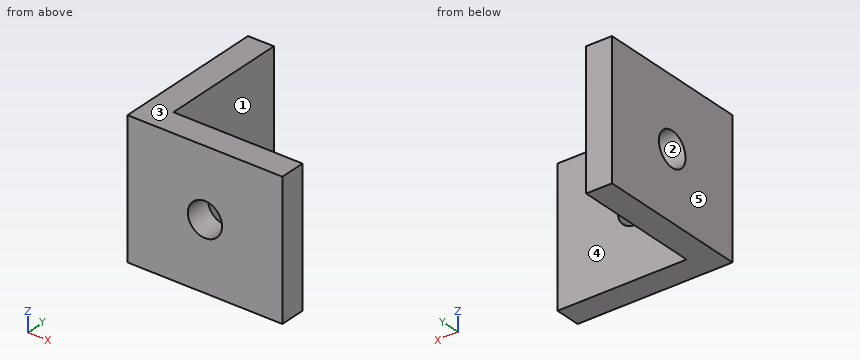
from build123d import *

# Parameters (mm, degrees)
BODY_DEPTH   = 33.27
SKETCH2_R    = 4.2
HOLESX_DEPTH = 6.35
SKETCH3_R    = 4.2
HOLESY_DEPTH = 6.35


with BuildPart() as part:
    # Sketch1 → Body (new body)
    with BuildSketch(Plane.XY.offset(-16.635)):
        Polygon((0, 0), (38.1, 0), (38.1, 6.35), (6.35, 6.35), (6.35, 38.1), (0, 38.1), align=None)
    extrude(amount=BODY_DEPTH)

    # Sketch2 → HolesX (cut)
    with BuildSketch(Plane(origin=(0, 6.35, 0), x_dir=(1, 0, 0), z_dir=(0, 1, 0))):
        with Locations(Location((19.05, 0, 0), (0, 0, 270))):
            Circle(SKETCH2_R)
    extrude(amount=-HOLESX_DEPTH, mode=Mode.SUBTRACT)

    # Sketch3 → HolesY (cut)
    with BuildSketch(Plane(origin=(6.35, 0, 0), x_dir=(0, 0, -1), z_dir=(1, 0, 0))):
        with Locations((0, 19.05)):
            Circle(SKETCH3_R)
    extrude(amount=-HOLESY_DEPTH, mode=Mode.SUBTRACT)


solid = part.part
Geometry check sheet. Reference: the model listing, model coordinates, mm. Face numbers are marked on the shaded views. A direction names the side the tool comes from. Coordinates: 2 decimals unless noted, no trailing zeros. Order: outer loops, then holes, each group sorted by start corner. A loop starts at its lowest first (then second) coordinate and runs counter-clockwise, first axis right, second up. Notation, with made-up numbers: (82.25, 74.25) - (94.25, 74.25) arc R17 ccw to (94.25, 89.25) - close; hole circle Ø3 at (33, 65.5). An arc over 180 degrees is marked (long way). One line per item, written item: value.
(1) Sectioned sample at C-C (z = 0). Enter the section's corners in (x, y), and give its area (3 significant figures).
Data:
outline: (0, 0) - (14.85, 0) - (14.85, 6.35) - (6.35, 6.35) - (6.35, 14.85) - (0, 14.85) - close; (0, 23.25) - (6.35, 23.25) - (6.35, 38.1) - (0, 38.1) - close; (23.25, 0) - (38.1, 0) - (38.1, 6.35) - (23.25, 6.35) - close
area: 337 mm^2
(2) Release check for a two-part mould opening along Z. For the marked faces 1, 2 and 3 record: +Z half, -Z half, draft (parallel to the pull), parting line (faces both ways), or undercut.
Data:
face 1: draft
face 2: undercut
face 3: +Z half
(3) Sectioned sample at A-A (y = 19.05). Enter the section's corners in (x, z) (3 decimals).
Data:
outline: (0, -16.635) - (6.35, -16.635) - (6.35, -4.2) - (0, -4.2) - close; (0, 4.2) - (6.35, 4.2) - (6.35, 16.635) - (0, 16.635) - close
(4) Thickness scan on probe 1 along X at (y, z) = (2.5, 0); probe 2 along Z at (x, y) = (1, 19) (3 decimals). Record the ranges inside material, lowest first. Write a range as from..to.
Data:
probe 1: x = 0..14.85, 23.25..38.1
probe 2: z = -16.635..-4.2, 4.2..16.635
(5) Sectioned sample at D-D (y = 7). Enter the section's corners in (x, z) (3 decimals).
Data:
outline: (0, -16.635) - (6.35, -16.635) - (6.35, 16.635) - (0, 16.635) - close
(6) Access from +Z, -Z, +X, -X, +Y, -Y to the whole of each face (thin tool, end or side, straight path). Record for the marked faces 4 and 5.
Data:
face 4: +Z, -Z, +X, +Y
face 5: +Z, -Z, -X, +Y, -Y
(7) Depth check by flat-ended pin: pin 1 Ø11 at (y, z) = (19.05, 0) entering from +X. Enter the tip coordinate at first touch or a pass-through.
Data:
pin 1: stops at x = 6.35
